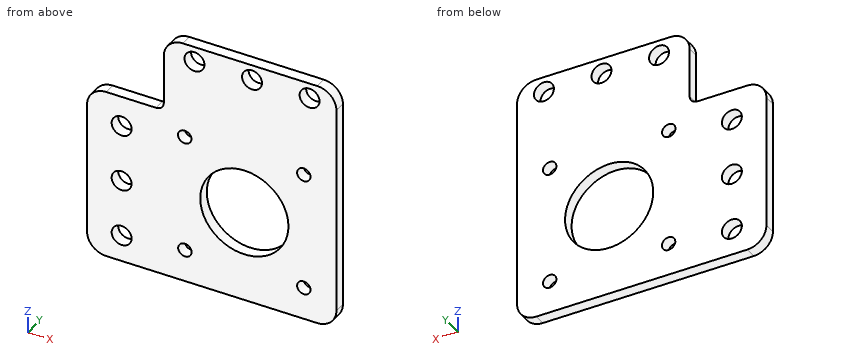
```python
from build123d import *

# Parameters (mm, degrees)
SKETCH2_R          = 2.6
SKETCH2_R_2        = 1.75
SKETCH2_R_3        = 11.5
BASE_FLANGE1_DEPTH = 3
FILLET1_R          = 5
FILLET2_R          = 2


# Sheet-metal steps are written as plain solids
with BuildPart() as part:
    # Sketch2 → Base-Flange1 (new body)
    with BuildSketch(Plane(origin=(0, 0, 0), x_dir=(1, 0, 0), z_dir=(0, 1, 0))):
        Polygon((0, 70), (65, 70), (65, 5), (20, 5), (20, 25), (0, 25), align=None)
        with Locations(Location((28, 9, 0), (0, 0, 270))):
            Circle(SKETCH2_R, mode=Mode.SUBTRACT)
        with Locations(Location((43, 9, 0), (0, 0, 270))):
            Circle(SKETCH2_R, mode=Mode.SUBTRACT)
        with Locations(Location((58, 9, 0), (0, 0, 270))):
            Circle(SKETCH2_R, mode=Mode.SUBTRACT)
        with Locations(Location((9, 33, 0), (0, 0, 270))):
            Circle(SKETCH2_R, mode=Mode.SUBTRACT)
        with Locations(Location((9, 48, 0), (0, 0, 270))):
            Circle(SKETCH2_R, mode=Mode.SUBTRACT)
        with Locations(Location((9, 63, 0), (0, 0, 270))):
            Circle(SKETCH2_R, mode=Mode.SUBTRACT)
        with Locations(Location((25.5, 61.5, 0), (0, 0, 270))):
            Circle(SKETCH2_R_2, mode=Mode.SUBTRACT)
        with Locations(Location((56.5, 61.5, 0), (0, 0, 270))):
            Circle(SKETCH2_R_2, mode=Mode.SUBTRACT)
        with Locations(Location((56.5, 30.5, 0), (0, 0, 270))):
            Circle(SKETCH2_R_2, mode=Mode.SUBTRACT)
        with Locations(Location((25.44917982, 30.502293897, 0), (0, 0, 270))):
            Circle(SKETCH2_R_2, mode=Mode.SUBTRACT)
        with Locations(Location((41, 46, 0), (0, 0, 270))):
            Circle(SKETCH2_R_3, mode=Mode.SUBTRACT)
    extrude(amount=-BASE_FLANGE1_DEPTH)

    # Fillet1
    fillet1_edges = [part.edges().sort_by_distance(p)[0] for p in [
        (0, -1.5, -25),
        (0, -1.5, -70),
        (65, -1.5, -70),
        (65, -1.5, -5),
        (20, -1.5, -5),
    ]]
    fillet(fillet1_edges, radius=FILLET1_R)

    # Fillet2
    fillet2_edges = [part.edges().sort_by_distance(p)[0] for p in [
        (20, -1.5, -25),
    ]]
    fillet(fillet2_edges, radius=FILLET2_R)


solid = part.part
```
Input: part model. Units: mm. Frame: model coordinates. Give positions to 0.01 mm unless a question says otherwise; leave off trailing zeros. Order: outer loops, then holes, each group sorted by start corner. A loop starts at its lowest first (then second) coordinate and runs counter-clockwise, first axis right, second up. Notation, with made-up numbers: (-10, 49) - (34, 49) arc R17 cw to (34, 57) - close; hole circle Ø8 at (68.5, 57). An arc over 180 degrees is marked (long way). Use a Markdown table: item, result.
(1) Section query A-A (x = 28). Output: boundary loops of the cut face in (y, z).
Computed values:
| item | result |
|---|---|
| outline | (-3, -70) - (0, -70) - (0, -11.6) - (-3, -11.6) - close; (-3, -6.4) - (0, -6.4) - (0, -5) - (-3, -5) - close |
(2) Line query: line 1 (X direction, y = -0.9, z = -46); line 2 (X direction, y = -0.95, z = -9); line 3 (X direction, y = -2.4, z = -33). Output: solid intervals per line, ascending. Write a range as from..to.
Computed values:
| item | result |
|---|---|
| line 1 | x = 0..7.34, 10.66..29.5, 52.5..65 |
| line 2 | x = 20.1..25.4, 30.6..40.4, 45.6..55.4, 60.6..64.9 |
| line 3 | x = 0..6.4, 11.6..65 |
(3) Section query B-B (z = -33). Output: boundary loops of the cut face in (x, y).
Computed values:
| item | result |
|---|---|
| outline | (0, -3) - (6.4, -3) - (6.4, 0) - (0, 0) - close; (11.6, -3) - (65, -3) - (65, 0) - (11.6, 0) - close |
(4) Section query D-D (z = -9). Output: boundary loops of the cut face in (x, y), then the cut area to 3 significant figures.
Computed values:
| item | result |
|---|---|
| outline | (20.1, -3) - (25.4, -3) - (25.4, 0) - (20.1, 0) - close; (30.6, -3) - (40.4, -3) - (40.4, 0) - (30.6, 0) - close; (45.6, -3) - (55.4, -3) - (55.4, 0) - (45.6, 0) - close; (60.6, -3) - (64.9, -3) - (64.9, 0) - (60.6, 0) - close |
| area | 87.6 mm2 |
(5) Section query C-C (x = 9). Output: boundary loops of the cut face in (y, z), then the cut area to 3 significant figures.
Computed values:
| item | result |
|---|---|
| outline | (-3, -70) - (0, -70) - (0, -65.6) - (-3, -65.6) - close; (-3, -60.4) - (0, -60.4) - (0, -50.6) - (-3, -50.6) - close; (-3, -45.4) - (0, -45.4) - (0, -35.6) - (-3, -35.6) - close; (-3, -30.4) - (0, -30.4) - (0, -25) - (-3, -25) - close |
| area | 88.2 mm2 |
